```python
from build123d import *

# Parameters (mm, degrees)
F0_W     = 600
F0_H     = 100
F1_DEPTH = 100
F3_DEPTH = 100.001
F4_DEPTH = 100.001


with BuildPart() as f1:
    # F0 (on Front) → F1 (new body)
    with BuildSketch(Plane.XZ):
        Rectangle(F0_W, F0_H)
    extrude(amount=F1_DEPTH)

    # F2 (on face) → F3 (cut, through all)
    with BuildSketch(Plane.XY.offset(50)):
        Polygon((-200, -100), (-300, 0), (-300, -100), align=None)
    extrude(amount=-F3_DEPTH, mode=Mode.SUBTRACT)

    # F2 (on face) → F4 (cut, through all)
    with BuildSketch(Plane.XY.offset(50)):
        Polygon((300, -100), (300, 0), (200, -100), align=None)
    extrude(amount=-F4_DEPTH, mode=Mode.SUBTRACT)


solid = f1.part
```
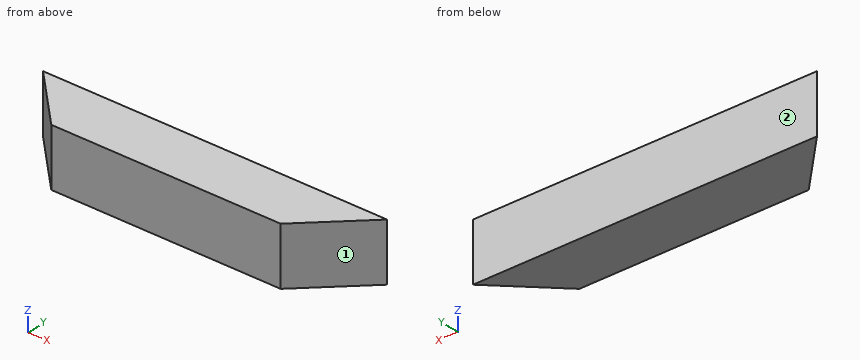
Build history of the part. All positions in model axes, mm. Face numbers are marked on the shaded views. Round coordinates to 2 decimals unless told otherwise and drop trailing zeros. Order: outer loops, then holes, each group sorted by start corner. A loop starts at its lowest first (then second) coordinate and runs counter-clockwise, first axis right, second up. Notation, with made-up numbers: (-38.5, 34) -> (13.5, 34) arc R10 cw to (13.5, 43) -> close; hole circle Ø10 at (29, -6). An arc over 180 degrees is marked (long way). Answer in a Markdown table with one row per item.
1) Pin check, flat tips, straight feed: P1, Ø5, axis at y = -64, z = -22.5, coming from the +X side; P2, Ø5, axis at y = -69, z = 11.5, coming from the +X side; P3, Ø2, axis at y = -77, z = 25.5, coming from the +X side. Stop position of each tip, or through.
Values:
| item | result |
|---|---|
| P1 | x = 238.5 |
| P2 | x = 233.5 |
| P3 | x = 224 |
2) Wall check: L1, parallel to X at y = -75, z = -14; L2, parallel to X at y = -41, z = 23; L3, parallel to Y at x = -245.5, z = 33.5. Give the ranges that are in metal, low to high.
Values:
| item | result |
|---|---|
| L1 | -225 to 225 |
| L2 | -259 to 259 |
| L3 | -54.5 to 0 |
3) Band-saw the part on B-B on y = -61. Give the cut face in (x, z).
Values:
| item | result |
|---|---|
| outline | (-239, -50) -> (239, -50) -> (239, 50) -> (-239, 50) -> close |
4) Mould opens along X. For the marked faces 1 and 2 say: released by +X, released by -X, zero draft, split by the parting line, or undercut.
Values:
| item | result |
|---|---|
| face 1 | released by +X |
| face 2 | zero draft |
5) Band-saw the part on A-A on z = -6. Give the cut face in (x, y), and give its area (3 significant figures).
Values:
| item | result |
|---|---|
| outline | (-300, 0) -> (-200, -100) -> (200, -100) -> (300, 0) -> close |
| area | 50,000 mm2 |
